```python
from build123d import *

# Parameters (mm, degrees)
PAD005_DEPTH    = 12
POCKET003_DEPTH = 4.5
SKETCH012_R     = 1.7
HOLE003_DEPTH   = 25


with BuildPart() as part:
    # Sketch010 → Pad005 (new body)
    with BuildSketch(Plane.XY):
        Polygon((0, 0), (0, 8), (-4, 8), (-7.9, 4.1), (-7.9, 2.2), (-3.75, 2.2), (-3.75, 0), align=None)
    pad005 = extrude(amount=PAD005_DEPTH)

    # Mirrored003: Pad005 across Sketch010 V_Axis
    add(pad005.mirror(Plane(origin=(0, 0, 0), x_dir=(0, 0, 1), z_dir=(1, 0, 0))))

    # Sketch011 (on DatumPlane) → Pocket003 (cut)
    with BuildSketch(Plane(origin=(0, 8, 0), x_dir=(-1, 0, 0), z_dir=(0, 1, 0))):
        Polygon((0, 2.535898), (3, 4.267949), (3, 7.732051), (0, 9.464102), (-3, 7.732051), (-3, 4.267949), align=None)
    extrude(amount=-POCKET003_DEPTH, mode=Mode.SUBTRACT)

    # Sketch012 (on DatumPlane) → Hole003 (cut)
    with BuildSketch(Plane(origin=(0, 8, 0), x_dir=(-1, 0, 0), z_dir=(0, 1, 0))):
        with Locations((0, 6)):
            Circle(SKETCH012_R)
    extrude(amount=-HOLE003_DEPTH, mode=Mode.SUBTRACT)


solid = part.part
```
Can you work these out from the model? Positions are in its coordinate system, mm. A direction names the side the tool comes from. Give positions to 0.01 mm unless a question says otherwise; leave off trailing zeros. Loops run counter-clockwise (first coordinate to the right, second up) from the corner with the lowest first, then second, coordinate; pieces in that order, holes last. Notation, with made-up numbers: M -6,82.5 L 40,82.5 A6 ccw 40,88.5 Z; hole C 52.5,-36.75 d4. An arc over 180 degrees is marked long. One line per question, with ' | ' between items. Start each with the question number.
Q1. If we section it at D-D (x = -2.25): Please give me the cut outline in (y, z).
Q2. If I drill on line 1 (Z direction, x = 0, y = 1.15); line 2 (X direction, y = 3.75, z = 3.75); line 3 (Z direction, x = 1, y = 7), over which ranges is the centre line in solid material (lowest first)? Write a range as from..to.
Q3. If we section it at C-C (z = 1.25): Please give me the cut outline in (x, y), plus the area to 3 significant figures.
Q4. For pin 1 Ø1.1 at (y, z) = (1, 3.5) entering from +X; pin 2 Ø2 at (x, z) = (-6.5, 5) entering from -Y; pin 3 Ø4 at (y, z) = (7, 8.5) entering from +X, each with a flat end and sliding along its axis, tell me the tip position at first contact or that it passes through.
Q5. If we section it at B-B (z = 6): Please give me the cut outline in (x, y).
Q6. For faces 1 (the flat face through (1.5, 5.8, 3.4)), 2 (the flat face through (-3.75, 1, 6)), 3 (the flat face through (6, 2.2, 6)), which set-ups out of +Z, -Z, +X, -X, +Y, -Y let a thin tool reach every point of the face, with its end or its side?
Q7. If we mould it in two halves opening along X, with no side actions, what happens to faces 4 (the flat face through (1, 3.5, 8)), 5 (the flat face through (-6, 6, 6)), 6 (the flat face through (-6, 2.2, 6))? For each: +X half, -X half, draft (parallel to the pull), parting line (faces both ways), or undercut.
Q8. If we section it at A-A (y = 6.5): Please give me the cut outline in (x, z), plus the area to 3 significant figures.
Computed:
1) outline: M 0,0 L 8,0 L 8,3.83 L 3.5,3.83 L 3.5,8.17 L 8,8.17 L 8,12 L 0,12 Z
2) line 1: z = 0..4.3, 7.7..12 | line 2: x = -7.9..-2.1, 2.1..7.9 | line 3: z = 0..3.11, 8.89..12
3) outline: M -7.9,2.2 L -3.75,2.2 L -3.75,0 L 3.75,0 L 3.75,2.2 L 7.9,2.2 L 7.9,4.1 L 4,8 L -4,8 L -7.9,4.1 Z | area: 92.9 mm²
4) pin 1: stops at x = 3.75 | pin 2: stops at y = 2.2 | pin 3: stops at x = 7
5) outline: M -7.9,2.2 L -3.75,2.2 L -3.75,0 L -1.7,0 L -1.7,3.5 L -3,3.5 L -3,8 L -4,8 L -7.9,4.1 Z; M 1.7,0 L 3.75,0 L 3.75,2.2 L 7.9,2.2 L 7.9,4.1 L 4,8 L 3,8 L 3,3.5 L 1.7,3.5 Z
6) face 1: +Y | face 2: +Z, -Z, -X, -Y | face 3: +Z, -Z, +X, -Y
7) face 4: undercut | face 5: -X half | face 6: draft
8) outline: M -5.5,0 L 5.5,0 L 5.5,12 L -5.5,12 Z; hole M -3,4.27 L 0,2.54 L 3,4.27 L 3,7.73 L 0,9.46 L -3,7.73 Z | area: 101 mm²
